```python
from build123d import *

# Parameters (mm, degrees)
F0_W     = 4.7625
F0_H     = 4.7625
F1_DEPTH = 9.525
F3_DEPTH = 25.4
F5_DEPTH = 25.4
F6_R     = 1.8034
F7_DEPTH = 9.525


with BuildPart() as f1:
    # F0 (on Front) → F1 (new body)
    with BuildSketch(Plane.XZ):
        Rectangle(F0_W, F0_H)
    extrude(amount=F1_DEPTH)

    # F2 (on face) → F3 (cut)
    with BuildSketch(Plane.XY.offset(2.38125)):
        Polygon((-0.79375, -9.525), (0, -9.525), (0.79375, -9.525), (0.79375, -7.9375), (-0.79375, -7.9375), align=None)
    extrude(amount=-F3_DEPTH, mode=Mode.SUBTRACT)

    # F4 (on face) → F5 (cut)
    with BuildSketch(Plane(origin=(0, 0, 0), x_dir=(-1, 0, 0), z_dir=(0, 1, 0))):
        with BuildLine():
            ThreePointArc((-2.38125, 0), (-1.6837980227, 1.6837980227), (0, 2.38125))
            Line((0, 2.38125), (-2.38125, 2.38125))
            Line((-2.38125, 2.38125), (-2.38125, 0))
        make_face()
        with BuildLine():
            ThreePointArc((0, 2.38125), (1.6837980227, 1.6837980227), (2.38125, 0))
            Line((2.38125, 0), (2.38125, 2.38125))
            Line((2.38125, 2.38125), (0, 2.38125))
        make_face()
        with BuildLine():
            Line((2.38125, -2.38125), (2.38125, 0))
            ThreePointArc((2.38125, 0), (1.6837980227, -1.6837980227), (0, -2.38125))
            Line((0, -2.38125), (2.38125, -2.38125))
        make_face()
        with BuildLine():
            Line((-2.38125, -2.38125), (0, -2.38125))
            ThreePointArc((0, -2.38125), (-1.6837980227, -1.6837980227), (-2.38125, 0))
            Line((-2.38125, 0), (-2.38125, -2.38125))
        make_face()
    extrude(amount=-F5_DEPTH, mode=Mode.SUBTRACT)

    # F6 (on face) → F7 (join)
    with BuildSketch(Plane(origin=(0, 0, 0), x_dir=(-1, 0, 0), z_dir=(0, 1, 0))):
        Circle(F6_R)
    extrude(amount=F7_DEPTH)


solid = f1.part
```
Source: CAD feature listing. Evaluate the final solid. Frame: model axes, mm. A direction names the side the tool comes from. Give positions to 0.01 mm unless a question says otherwise; leave off trailing zeros. Order: outer loops, then holes, each group sorted by start corner. A loop starts at its lowest first (then second) coordinate and runs counter-clockwise, first axis right, second up. Notation, with made-up numbers: (25, 87.5) -> (55, 87.5) arc R27 cw to (55, 121.5) -> close; hole circle Ø6 at (42.5, 86). An arc over 180 degrees is marked (long way). Use a Markdown table: item, result.
Q1. First-contact query: P1, Ø1, axis at x = 0.5, y = -6, coming from the +Z side; P2, Ø1, axis at y = 2, z = 2, coming from the +X side; P3, Ø1.5, axis at x = 1, y = 3, coming from the +Z side; P4, Ø0.5, axis at y = -9, z = 0.5, coming from the -X side. Flat tips, straight axial feed; report the tip coordinate or a pass-through.
A:
| item | result |
|---|---|
| P1 | z = 2.38 |
| P2 | x = 1 |
| P3 | z = 1.79 |
| P4 | x = -2.37 |
Q2. Section C-C (y = 5). Return the cut outline in (x, z), and give its area (3 significant figures).
A:
| item | result |
|---|---|
| outline | circle Ø3.61 at (0, 0) |
| area | 10.2 mm^2 |
Q3. Section D-D (z = 1.6). Return the cut outline in (x, y) (1 decimal).
A:
| item | result |
|---|---|
| outline | (-1.8, -9.5) -> (-0.8, -9.5) -> (-0.8, -7.9) -> (0.8, -7.9) -> (0.8, -9.5) -> (1.8, -9.5) -> (1.8, 0) -> (0.8, 0) -> (0.8, 9.5) -> (-0.8, 9.5) -> (-0.8, 0) -> (-1.8, 0) -> close |
Q4. Section A-A (z = -0.5). Return the cut outline in (x, y) (1 decimal), and give its area (3 significant figures).
A:
| item | result |
|---|---|
| outline | (-2.3, -9.5) -> (-0.8, -9.5) -> (-0.8, -7.9) -> (0.8, -7.9) -> (0.8, -9.5) -> (2.3, -9.5) -> (2.3, 0) -> (1.7, 0) -> (1.7, 9.5) -> (-1.7, 9.5) -> (-1.7, 0) -> (-2.3, 0) -> close |
| area | 74.8 mm^2 |
Q5. Material intervals for line 1 (X direction, y = -3, z = 0.8); line 2 (Y direction, x = -0.25, z = 2.15); line 3 (X direction, y = -8.25, z = -1), sorted ascending. Write a range as [from, to].
A:
| item | result |
|---|---|
| line 1 | [-2.24, 2.24] |
| line 2 | [-7.94, 0] |
| line 3 | [-2.16, -0.79], [0.79, 2.16] |
Q6. Access query for faces 5 (the face through (0, -7.938, 0)), 6 (the face through (-1, -9.525, 0)), 7 (the face through (0, 0, 2)). Directions: +Z, -Z, +X, -X, +Y, -Y. A direction counts if a zero-diameter tool reaches every point of the face in a straight line with its end or side. Return the directions, or none.
A:
| item | result |
|---|---|
| face 5 | +Z, -Z, -Y |
| face 6 | +Z, -Z, +X, -X, -Y |
| face 7 | +Y |
Q7. Pull-direction query (X, two-part tool) for faces 1 (the face through (0, 9.525, 0)), 2 (the face through (0.794, -9, 0)), 3 (the face through (1.43, 4.7, -1.1)), 4 (the face through (-0.794, -9, 0)); classes: +X half, -X half, draft (parallel to the pull), parting line (faces both ways), or undercut.
A:
| item | result |
|---|---|
| face 1 | draft |
| face 2 | undercut |
| face 3 | parting line |
| face 4 | undercut |
Q8. Section B-B (x = -0.45). Return the cut outline in (y, z) (1 decimal).
A:
| item | result |
|---|---|
| outline | (-7.9, -2.3) -> (0, -2.3) -> (0, -1.7) -> (9.5, -1.7) -> (9.5, 1.7) -> (0, 1.7) -> (0, 2.3) -> (-7.9, 2.3) -> close |
